from build123d import *

# Parameters (mm, degrees)
SKETCH_2_R      = 4.5
SKETCH_2_R_2    = 2.15
EXTRUDE_1_DEPTH = 22
EXTRUDE_START   = -2
SKETCH_3_R      = 5.5
SKETCH_3_R_2    = 2.15
EXTRUDE_2_DEPTH = 2
CHAMFER_1_SIZE  = 1.5


with BuildPart() as part:
    # 草图2 → 凸台-拉伸1 (new, symmetric)
    with BuildSketch(Plane(origin=(0, 0, 0), x_dir=(1, 0, 0), z_dir=(0, 1, 0))):
        with Locations(Location((0, 0, 0), (0, 0, 270))):
            Circle(SKETCH_2_R)
        with Locations(Location((0, 0, 0), (0, 0, 270))):
            Circle(SKETCH_2_R_2, mode=Mode.SUBTRACT)
    extrude(amount=EXTRUDE_1_DEPTH, both=True)

    # 草图3 → 凸台-拉伸2 (add)
    with BuildSketch(Plane(origin=(0, 22, 0), x_dir=(1, 0, 0), z_dir=(0, 1, 0)).offset(EXTRUDE_START)):
        with Locations(Location((0, 0, 0), (0, 0, 270))):
            Circle(SKETCH_3_R)
        with Locations(Location((0, 0, 0), (0, 0, 270))):
            Circle(SKETCH_3_R_2, mode=Mode.SUBTRACT)
    extrude_2 = extrude(amount=EXTRUDE_2_DEPTH)

    # 镜向1: 凸台-拉伸2 across plane
    add(extrude_2.mirror(Plane.ZX))

    # 倒角1
    # the kernel refuses this chamfer: 1.5 mm, written as the material it adds along each edge
    with BuildSketch(Plane(origin=(0, -20, 0), x_dir=(0, 0, 1), z_dir=(-1, 0, 0))) as chamfer_1_piece_1_section:
        Polygon((4.5 + CHAMFER_1_SIZE, 0), (4.5, CHAMFER_1_SIZE), (4.5, 0), align=None)
    chamfer_1_piece_1 = revolve(axis=Axis((0, -20, 0), (0, 1, 0)), mode=Mode.PRIVATE)
    chamfer_1_piece_1 = chamfer_1_piece_1 & Plane(origin=(0, -19.001553526, 0), x_dir=(0, 0, 1), z_dir=(0, 1, 0)) * Cylinder(5.5, 24, mode=Mode.PRIVATE)
    add(chamfer_1_piece_1)
    with BuildSketch(Plane(origin=(0, 20, 0), x_dir=(0, 0, 1), z_dir=(-1, 0, 0))) as chamfer_1_piece_2_section:
        Polygon((4.5, -CHAMFER_1_SIZE), (4.5 + CHAMFER_1_SIZE, 0), (4.5, 0), align=None)
    chamfer_1_piece_2 = revolve(axis=Axis((0, 20, 0), (0, 1, 0)), mode=Mode.PRIVATE)
    chamfer_1_piece_2 = chamfer_1_piece_2 & Plane(origin=(0, 19.001553526, 0), x_dir=(0, 0, 1), z_dir=(0, -1, 0)) * Cylinder(5.5, 24, mode=Mode.PRIVATE)
    add(chamfer_1_piece_2)


solid = part.part
For this review, take the finished solid that the model builds, in its own axes (mm). A direction names the side the tool comes from. Give positions to 0.01 mm unless a question says otherwise; leave off trailing zeros. Loops run counter-clockwise (first coordinate to the right, second up) from the corner with the lowest first, then second, coordinate; pieces in that order, holes last.
Item 1: For line 1 along X through (y, z) = (5, 0); line 2 along Y through (x, z) = (4.5, 3); line 3 along Z through (x, y) = (-0.5, 10), list the stretches that pass through material, from the lowest coordinate up.
Item 2: Take a section at A-A, the plane x = 0. State the section outline as (y, z) points, and give its area (3 significant figures).
Item 3: Insertion check: pin 1 (1 mm diameter, centred on y = -7, z = -3.5, fed in from +X); pin 2 (1 mm diameter, centred on x = -1, y = 2.5, fed in from +Z); pin 3 (6 mm diameter, centred on y = -9.5, z = 1.5, fed in from +X). Each pin has a flat end and moves straight along its axis. Give the tip position at first contact, or say it passes through.
Item 4: Take a section at C-C, the plane y = 14. State the section outline as (x, z) points.
Item 5: Tool access review of faces 1 (the cylindrical face through (-5.37, -20.73, -1.19)), 2 (the cylindrical face through (1.352, 0.259, 4.292)): name each direction out of +Z, -Z, +X, -X, +Y, -Y from which nothing blocks a thin tool from reaching the whole face with its end or side.
Item 6: Draft analysis for pull direction Z (two halves, no side actions). For faces 3 (the cylindrical face through (5.37, 20.73, -1.19)), 4 (the cylindrical face through (-1.308, -0.308, -1.706)), 5 (the flat face through (-2.4, -22, -0.1)), state which applies: +Z half, -Z half, draft (parallel to the pull), parting line (faces both ways), or undercut.
Item 7: Take a section at B-B, the plane z = 0. State the section outline as (x, y) points.
Calculated:
1. line 1: x = -4.5 to -2.15, 2.15 to 4.5
1. line 2: y = -22 to -19.41, 19.41 to 22
1. line 3: z = -4.47 to -2.09, 2.09 to 4.47
2. outline: (-22, -5.5) - (-19.5, -5.5) - (-18.5, -4.5) - (18.5, -4.5) - (19.5, -5.5) - (22, -5.5) - (22, -2.15) - (-22, -2.15) - close; (-22, 2.15) - (22, 2.15) - (22, 5.5) - (19.5, 5.5) - (18.5, 4.5) - (-18.5, 4.5) - (-19.5, 5.5) - (-22, 5.5) - close
2. area: 219 mm2
3. pin 1: stops at x = 3.35
3. pin 2: stops at z = 4.47
3. pin 3: stops at x = 4.5
4. outline: circle Ø9 at (0, 0); hole circle Ø4.3 at (0, 0)
5. face 1: +Y, -Y
5. face 2: none
6. face 3: parting line
6. face 4: undercut
6. face 5: draft
7. outline: (-5.5, -22) - (-2.15, -22) - (-2.15, 22) - (-5.5, 22) - (-5.5, 19.5) - (-4.5, 18.5) - (-4.5, -18.5) - (-5.5, -19.5) - close; (2.15, -22) - (5.5, -22) - (5.5, -19.5) - (4.5, -18.5) - (4.5, 18.5) - (5.5, 19.5) - (5.5, 22) - (2.15, 22) - close
